```python
from build123d import *

# Parameters (mm, degrees)
F0_W     = 76.2
F0_H     = 101.6
F1_DEPTH = 25.4
F2_W     = 63.5
F2_H     = 19.05
F3_DEPTH = 76.2
F5_DEPTH = 54.60239
F6_DEPTH = 25.4
F8_D     = 12.7
F8_DEPTH = 215.9
F8_TIP   = 3.8154649308
F9_DEPTH = 25.4
F10_SIZE = 6.34999


# Not quite as in the source:
# - a fillet or chamfer is up to 0.001 mm smaller than in the source, because OpenCascade refuses the exact size


with BuildPart() as f1:
    # F0 (on Top) → F1 (new body)
    with BuildSketch(Plane.XY):
        with Locations((-6.5660695493, 0.5611634433)):
            Rectangle(F0_W, F0_H)
    extrude(amount=F1_DEPTH)

    # F2 (on face) → F3 (join)
    with BuildSketch(Plane.XY.offset(25.4)):
        with Locations((-6.5660695493, -8.9638365567)):
            Rectangle(F2_W, F2_H)
    extrude(amount=F3_DEPTH)

    # F4 (on face) → F5 (cut)
    with BuildSketch(Plane.XZ.offset(18.4888365567)):
        with BuildLine():
            Line((-38.3160695493, 101.6), (-38.3160695493, 63.5))
            ThreePointArc((-38.3160695493, 63.5), (-32.1637379002, 82.2835533113), (-16.0910695493, 93.787569645))
            Line((-16.0910695493, 93.787569645), (-16.0910695493, 101.6))
            Line((-16.0910695493, 101.6), (-38.3160695493, 101.6))
        make_face()
        with BuildLine():
            ThreePointArc((-16.0910695493, 93.787569645), (-6.5660695493, 95.25), (2.9589304507, 93.787569645))
            Line((2.9589304507, 93.787569645), (2.9589304507, 101.6))
            Line((2.9589304507, 101.6), (-16.0910695493, 101.6))
            Line((-16.0910695493, 101.6), (-16.0910695493, 93.787569645))
        make_face()
        with BuildLine():
            ThreePointArc((2.9589304507, 93.787569645), (19.0315988015, 82.2835533113), (25.1839304507, 63.5))
            Line((25.1839304507, 63.5), (25.1839304507, 101.6))
            Line((25.1839304507, 101.6), (2.9589304507, 101.6))
            Line((2.9589304507, 101.6), (2.9589304507, 93.787569645))
        make_face()
    extrude(amount=-F5_DEPTH, mode=Mode.SUBTRACT)

    # F4 (on face) → F6 (cut)
    with BuildSketch(Plane.XZ.offset(18.4888365567)):
        with BuildLine():
            Line((2.9589304507, 63.5), (2.9589304507, 93.787569645))
            ThreePointArc((2.9589304507, 93.787569645), (-6.5660695493, 95.25), (-16.0910695493, 93.787569645))
            Line((-16.0910695493, 93.787569645), (-16.0910695493, 63.5))
            ThreePointArc((-16.0910695493, 63.5), (-6.5660695493, 73.025), (2.9589304507, 63.5))
        make_face()
        with BuildLine():
            ThreePointArc((-16.0910695493, 63.5), (-13.3012616401, 56.7648079092), (-6.5660695493, 53.975))
            ThreePointArc((-6.5660695493, 53.975), (0.1691225415, 56.7648079092), (2.9589304507, 63.5))
            ThreePointArc((2.9589304507, 63.5), (-6.5660695493, 73.025), (-16.0910695493, 63.5))
        make_face()
    extrude(amount=-F6_DEPTH, mode=Mode.SUBTRACT)

    # F8
    with Locations(Plane.XY.offset(25.4)):
        with Locations((-28.7910695493, 35.4861634433), (15.6589304507, 35.4861634433), (15.6589304507, -34.3638365567), (-28.7910695493, -34.3638365567)):
            Hole(F8_D / 2, depth=F8_DEPTH)
            with Locations((0, 0, -(F8_DEPTH + F8_TIP / 2))):  # 118° drill point
                Cone(0, F8_D / 2, F8_TIP, mode=Mode.SUBTRACT)

    # F7 (on face) → F9 (cut)
    with BuildSketch(Plane.XY.offset(25.4)):
        with BuildLine():
            ThreePointArc((-44.6660695493, 35.4861634433), (-40.0163896548, 46.7114836405), (-28.7910694197, 51.3611634433))
            Line((-28.7910694197, 51.3611634433), (-44.6660695493, 51.3611634433))
            Line((-44.6660695493, 51.3611634433), (-44.6660695493, 35.4861634433))
        make_face()
        with BuildLine():
            Line((31.5339304507, 51.3611634433), (15.6589304507, 51.3611634433))
            ThreePointArc((15.6589304507, 51.3611634433), (26.884250602, 46.7114835947), (31.5339304507, 35.4861634433))
            Line((31.5339304507, 35.4861634433), (31.5339304507, 51.3611634433))
        make_face()
        with BuildLine():
            Line((31.5339304507, -50.2388365567), (31.5339304507, -34.3638365567))
            ThreePointArc((31.5339304507, -34.3638365567), (26.8842505737, -45.5891567363), (15.6589303706, -50.2388365567))
            Line((15.6589303706, -50.2388365567), (31.5339304507, -50.2388365567))
        make_face()
        with BuildLine():
            ThreePointArc((-28.7910695493, -50.2388365567), (-40.0163897007, -45.589156708), (-44.6660695493, -34.3638365567))
            Line((-44.6660695493, -34.3638365567), (-44.6660695493, -50.2388365567))
            Line((-44.6660695493, -50.2388365567), (-28.7910695493, -50.2388365567))
        make_face()
    extrude(amount=-F9_DEPTH, mode=Mode.SUBTRACT)

    # F10 (size 6.35 in the source; OpenCascade refuses exactly that, so slightly less here)
    f10_edges = [f1.edges().sort_by_distance(p)[0] for p in [
        (26.884251, -45.589157, 25.4),
        (31.53393, 0.561163, 25.4),
        (26.884251, 46.711484, 25.4),
        (-6.566069, 51.361163, 25.4),
        (-40.01639, 46.711484, 25.4),
        (-44.66607, 0.561163, 25.4),
        (-40.01639, -45.589157, 25.4),
        (-6.56607, -50.238837, 25.4),
    ]]
    chamfer(f10_edges, length=F10_SIZE)


solid = f1.part
```
Check sheet for the modelled part. Datum: model origin and axes. Units: mm. A direction names the side the tool comes from. Give positions to 0.01 mm unless a question says otherwise; leave off trailing zeros. Loops run counter-clockwise (first coordinate to the right, second up) from the corner with the lowest first, then second, coordinate; pieces in that order, holes last. Notation, with made-up numbers: M 35.25,88.5 L 75.25,88.5 A27 ccw 75.25,109.5 Z; hole C 31.5,77 d5. An arc over 180 degrees is marked long. Answer in a Markdown table with one row per item.
1) Cross-section at B-B (z = 87). Enter the section's corners in (x, y).
Solutions:
| item | result |
|---|---|
| outline | M -27.92,-18.49 L -16.09,-18.49 L -16.09,0.56 L -27.92,0.56 Z; M 2.96,-18.49 L 14.78,-18.49 L 14.78,0.56 L 2.96,0.56 Z |
2) Tool access check on faces 1 (the face through (-7, 0.561, 52)), 2 (the face through (-6.25, -47.11, 22.18)), 3 (the face through (2.959, -9, 78)). Record the directions out of +Z, -Z, +X, -X, +Y, -Y that give a thin tool (end or side, any length) a straight path to the whole face; none if there is none.
Solutions:
| item | result |
|---|---|
| face 1 | +Z, +X, -X, +Y |
| face 2 | +Z, +X, -X, -Y |
| face 3 | +Z, +Y, -Y |
3) Depth check by flat-ended pin: pin 1 (10 mm diameter, centred on y = -26, z = 43, fed in from -X); pin 2 (1 mm diameter, centred on x = 22.5, z = 36.5, fed in from +Y); pin 3 (21 mm diameter, centred on y = -5, z = 39, fed in from +X); pin 4 (20.5 mm diameter, centred on x = 15.66, y = -34.36, fed in from +Z). Enter the tip coordinate at first touch or a pass-through.
Solutions:
| item | result |
|---|---|
| pin 1 | passes through |
| pin 2 | stops at y = 0.56 |
| pin 3 | stops at x = 25.18 |
| pin 4 | stops at z = 25.4 |
4) Cross-section at D-D (x = 7.5). Enter the section's corners in (y, z), plus the area to 3 significant figures.
Solutions:
| item | result |
|---|---|
| outline | M -50.24,0 L 51.36,0 L 51.36,19.05 L 45.01,25.4 L 0.56,25.4 L 0.56,91.96 L -18.49,91.96 L -18.49,25.4 L -43.89,25.4 L -50.24,19.05 Z |
| area | 3,810 mm^2 |
5) Thickness scan on line 1 (Y direction, x = -29, z = 13); line 2 (Y direction, x = 16.5, z = 6.5); line 3 (Z direction, x = 19.5, y = 11). Record the ranges inside material, lowest first.
Solutions:
| item | result |
|---|---|
| line 1 | y = -50.24 to -40.71, -28.02 to 29.14, 41.83 to 51.36 |
| line 2 | y = -50.22 to -40.66, -28.07 to 29.19, 41.78 to 51.34 |
| line 3 | z = 0 to 25.4 |
6) Cross-section at C-C (y = -22). Enter the section's corners in (x, z).
Solutions:
| item | result |
|---|---|
| outline | M -44.67,0 L 31.53,0 L 31.53,19.05 L 25.18,25.4 L -38.32,25.4 L -44.67,19.05 Z |
7) Mould release check, pull along Y, two halves, no side actions. Record for faces 4 (the face through (-34.85, 37.39, 12.52)), 5 (the face through (-16.091, -9, 79)), 6 (the face through (24.078, 44.092, 22.886)), 7 (the face through (24.26, -42.78, 22.89)): released by +Y, released by -Y, zero draft, split by the parting line, or undercut.
Solutions:
| item | result |
|---|---|
| face 4 | undercut |
| face 5 | zero draft |
| face 6 | released by +Y |
| face 7 | released by -Y |
8) Cross-section at A-A (z = 7). Enter the section's corners in (x, y) (3 decimals), plus the area to 3 significant figures.
Solutions:
| item | result |
|---|---|
| outline | M -44.666,-34.364 A15.875 ccw -28.791,-50.239 L 15.659,-50.239 A15.875 ccw 31.534,-34.364 L 31.534,35.486 A15.875 ccw 15.659,51.361 L -28.791,51.361 A15.875 ccw -44.666,35.486 Z; hole C -28.791,-34.364 d12.7; hole C -28.791,35.486 d12.7; hole C 15.659,-34.364 d12.7; hole C 15.659,35.486 d12.7 |
| area | 7,020 mm^2 |
